Input: part model. Units: mm. Frame: model coordinates. A direction names the side the tool comes from. Round coordinates to 2 decimals unless told otherwise and drop trailing zeros. Loops run counter-clockwise (first coordinate to the right, second up) from the corner with the lowest first, then second, coordinate; pieces in that order, holes last.
(1) First-contact query: pin 1 Ø14.5 at (x, y) = (6, -152) entering from -Z; pin 2 Ø3 at (y, z) = (-139.5, -5.5) entering from +X; pin 3 Ø8 at (x, y) = (23.5, -156) entering from +Z. Flat tips, straight axial feed; report the tip coordinate or a pass-through.
(2) Cut plane C-C, the plane x = 23. Output: boundary loops of the cut face in (y, z), and give its area (3 significant figures).
(3) Line query: line 1 (Z direction, x = -3, y = -126); line 2 (X direction, y = -156, z = -7); line 3 (Y direction, x = -23.5, z = -7.25). Output: solid intervals per line, ascending.
(4) Draft query along Y for faces 5 (the face through (15.32, -131.41, 20.15)), 6 (the face through (-23.891, -153.026, -5.944)), 7 (the face through (0, -125, 0)). Return one class per face: released by +Y, released by -Y, zero draft, split by the parting line, or undercut.
(5) Cut plane B-B, the plane z = 15. Output: boundary loops of the cut face in (x, y), and give its area (3 significant figures).
(6) Access query for faces 1 (the face through (2.3, -61.76, 5.54)), 2 (the face through (0, 2, 12.5)), 3 (the face through (24.247, -144.084, -6.056)), 4 (the face through (0, -131, 9.9)). Directions: +Z, -Z, +X, -X, +Y, -Y. A direction counts if a zero-diameter tool reaches every point of the face in a straight line with its end or side. Return the directions, or none.
(7) Cut plane A-A, the plane y = -156. Output: boundary loops of the cut face in (x, z).
(8) Cut plane D-D, the plane x = -13.5. Output: boundary loops of the cut face in (y, z).
from build123d import *

# Parameters (mm, degrees)
SKETCH_1_W           = 52
SKETCH_1_H           = 25
SKETCH_1_R           = 1.5
EXTRUDE_1_DEPTH      = 5
SKETCH_2_R           = 4
SKETCH_2_R_2         = 2.5
EXTRUDE_2_DEPTH      = 125
FILLET_1_R           = 10
SKETCH_2_3_R         = 6
SKETCH_2_3_R_2       = 4
EXTRUDE_4_DEPTH      = 125
FILLET_3_R           = 5
CUT_EXTRUDE_START    = -50
SKETCH_2_4_R         = 6
CUT_EXTRUDE_1_DEPTH  = 50
FILLET_4_R           = 5
EXTRUDE_5_DEPTH      = 23
EXTRUDE_5_DEPTH_BACK = 10
SKETCH_3_W           = 36.659715442
SKETCH_3_H           = 13
SKETCH_4_W           = 12.2
SKETCH_4_H           = 10.2
CUT_EXTRUDE_2_DEPTH  = 16
FILLET_5_R           = 10
EXTRUDE_6_DEPTH      = 8
FILLET_9_R           = 5
SKETCH_10_W          = 42
SKETCH_10_H          = 8
EXTRUDE_7_DEPTH      = 3
SKETCH_8_R           = 3
CUT_EXTRUDE_5_DEPTH  = 179.328348954


with BuildPart() as part:
    # 草图1 → 凸台-拉伸1 (new body)
    with BuildSketch(Plane(origin=(0, 0, 0), x_dir=(1, 0, 0), z_dir=(0, 1, 0))):
        Rectangle(SKETCH_1_W, SKETCH_1_H)
        with Locations(Location((-18.5, 0, 0), (0, 0, 270))):
            Circle(SKETCH_1_R, mode=Mode.SUBTRACT)
        with Locations(Location((18.5, 0, 0), (0, 0, 270))):
            Circle(SKETCH_1_R, mode=Mode.SUBTRACT)
    extrude(amount=EXTRUDE_1_DEPTH)

    # 草图2 → 凸台-拉伸2 (add)
    with BuildSketch(Plane.XZ):
        with Locations(Location((0, 0, 0), (0, 0, 90))):
            Circle(SKETCH_2_R)
        with Locations(Location((0, 0, 0), (0, 0, 270))):
            Circle(SKETCH_2_R_2, mode=Mode.SUBTRACT)
    extrude(amount=EXTRUDE_2_DEPTH)

    # 圆角1
    fillet_1_edges = [part.edges().sort_by_distance(p)[0] for p in [
        (26, 2.5, 12.5),
        (-26, 2.5, 12.5),
        (-26, 2.5, -12.5),
        (26, 2.5, -12.5),
    ]]
    fillet(fillet_1_edges, radius=FILLET_1_R)

    # 草图2<3> → 凸台-拉伸4 (add)
    with BuildSketch(Plane.XZ):
        with Locations(Location((0, 0, 0), (0, 0, 90))):
            Circle(SKETCH_2_3_R)
        Circle(SKETCH_2_3_R_2, mode=Mode.SUBTRACT)
    extrude(amount=EXTRUDE_4_DEPTH)

    # 圆角3
    fillet_3_edges = [part.edges().sort_by_distance(p)[0] for p in [
        (0, 0, -6),
    ]]
    fillet(fillet_3_edges, radius=FILLET_3_R)

    # 草图2<4> → 切除-拉伸1 (cut)
    with BuildSketch(Plane.XZ.offset(CUT_EXTRUDE_START)):
        with Locations(Location((0, 0, 0), (0, 0, 90))):
            Circle(SKETCH_2_4_R)
    extrude(amount=CUT_EXTRUDE_1_DEPTH, mode=Mode.SUBTRACT)

    # 圆角4
    # the kernel refuses this fillet: 5 mm, written as the material it adds along each edge
    with BuildSketch(Plane(origin=(0, 0, 0), x_dir=(0, 0, 1), z_dir=(1, 0, 0))) as fillet_4_piece_1:
        with BuildLine():
            CenterArc((1, -4.769696007), FILLET_4_R, 0, 72.542396876)
            Line((2.5, 0), (2.53, 0.09539392))
            ThreePointArc((2.53, 0.09539392), (4.25, 0.1), (6, 0.1))
            Line((6, 0.1), (6.1, 0))
            Line((6.1, 0), (6.1, -4.769696007))
            Line((6.1, -4.769696007), (6, -4.769696007))
        make_face()
    revolve(axis=Axis((0, 0, 0), (0, -1, 0)))

    # 草图3 → 凸台-拉伸5 (add, two sides: drawn at the far end of the back side and taken through both)
    with BuildSketch(Plane.XY.offset(-EXTRUDE_5_DEPTH_BACK)):
        with Locations((0, -131.5)):
            Rectangle(SKETCH_3_W, SKETCH_3_H)
    extrude(amount=EXTRUDE_5_DEPTH + EXTRUDE_5_DEPTH_BACK)

    # 草图4 → 切除-拉伸2 (cut)
    with BuildSketch(Plane(origin=(0, -125, 0), x_dir=(1, 0, 0), z_dir=(0, 1, 0))):
        with Locations((0, -15)):
            Rectangle(SKETCH_4_W, SKETCH_4_H)
    extrude(amount=-CUT_EXTRUDE_2_DEPTH, mode=Mode.SUBTRACT)

    # 圆角5
    fillet_5_edges = [part.edges().sort_by_distance(p)[0] for p in [
        (18.329857721, -131.5, -10),
        (-18.329857721, -131.5, -10),
        (18.329857721, -131.5, 23),
        (-18.329857721, -131.5, 23),
    ]]
    fillet(fillet_5_edges, radius=FILLET_5_R)

    # 草图5 → 凸台-拉伸6 (add)
    with BuildSketch(Plane.XY.offset(-10)):
        Polygon((-18.329857721, -138), (-30, -150), (-30, -165), (-21, -174), (0, -174), (21, -174), (30, -165), (30, -150), (18.329857721, -138), align=None)
    extrude(amount=EXTRUDE_6_DEPTH)

    # 圆角9
    fillet_9_edges = [part.edges().sort_by_distance(p)[0] for p in [
        (0, -125, -6),
    ]]
    fillet(fillet_9_edges, radius=FILLET_9_R)

    # 草图10 → 凸台-拉伸7 (add)
    with BuildSketch(Plane.XZ.offset(174)):
        with Locations((0, -6)):
            Rectangle(SKETCH_10_W, SKETCH_10_H)
    extrude(amount=-EXTRUDE_7_DEPTH)

    # 草图8 → 切除-拉伸5 (cut, through all)
    with BuildSketch(Plane.XY.offset(-2)):
        with Locations((23.5, -156)):
            Circle(SKETCH_8_R)
        with Locations((-23.5, -156)):
            Circle(SKETCH_8_R)
    extrude(amount=-CUT_EXTRUDE_5_DEPTH, mode=Mode.SUBTRACT)


solid = part.part
Reported:
1. pin 1: stops at z = -10
1. pin 2: stops at x = 21.25
1. pin 3: stops at z = -2
2. outline: (-172, -10) - (-158.96, -10) - (-158.96, -2) - (-172, -2) - close; (-153.04, -10) - (-142.8, -10) - (-142.8, -2) - (-153.04, -2) - close; (0, -9.64) - (5, -9.64) - (5, 9.64) - (0, 9.64) - close
2. area: 283 mm2
3. line 1: z = -10 to 9.9, 20.1 to 23
3. line 2: x = -30 to -26.5, -20.5 to 20.5, 26.5 to 30
3. line 3: y = -171.5 to -159, -153 to -143.32, 0 to 5
4. face 5: zero draft
4. face 6: undercut
4. face 7: released by +Y
5. outline: (-18.13, -138) - (-6.1, -138) - (-6.1, -125) - (-18.13, -125) - close; (6.1, -138) - (18.13, -138) - (18.13, -125) - (6.1, -125) - close
5. area: 313 mm2
6. face 1: none
6. face 2: +Z, +X, -X, +Y
6. face 3: +Z, -Z, +X
6. face 4: -Y
7. outline: (-30, -10) - (-26.5, -10) - (-26.5, -2) - (-30, -2) - close; (-20.5, -10) - (20.5, -10) - (20.5, -2) - (-20.5, -2) - close; (26.5, -10) - (30, -10) - (30, -2) - (26.5, -2) - close
8. outline: (-174, -10) - (-138, -10) - (-138, -8.56) - (-125, -8.56) - (-125, 21.56) - (-138, 21.56) - (-138, -2) - (-174, -2) - close; (0, -12.5) - (5, -12.5) - (5, 12.5) - (0, 12.5) - close
